Check sheet for the modelled part. Datum: model origin and axes. Units: mm. A direction names the side the tool comes from. Round coordinates to 2 decimals unless told otherwise and drop trailing zeros. Loops run counter-clockwise (first coordinate to the right, second up) from the corner with the lowest first, then second, coordinate; pieces in that order, holes last. Notation, with made-up numbers: (9.5, 20) -> (15.5, 20) arc R19 ccw to (15.5, 47) -> close; hole circle Ø7 at (87.25, -37). An arc over 180 degrees is marked (long way). One line per question, with ' | ' between items.
```python
from build123d import *

# Parameters (mm, degrees)
SKETCH1_W           = 29
SKETCH1_H           = 28
SKETCH1_W_2         = 25
SKETCH1_H_2         = 13
BOSS_EXTRUDE1_DEPTH = 2
SKETCH2_R           = 1.45
CUT_EXTRUDE1_DEPTH  = 3
BOSS_EXTRUDE2_DEPTH = 29
SKETCH5_W           = 29
SKETCH5_H           = 2
BOSS_EXTRUDE3_DEPTH = 1
SKETCH6_W           = 2
SKETCH6_H           = 33
SKETCH6_H_2         = 1.6
BOSS_EXTRUDE4_DEPTH = 3
SKETCH7_W           = 2
SKETCH7_H           = 33
SKETCH7_H_2         = 1.6
BOSS_EXTRUDE5_DEPTH = 3


with BuildPart() as part:
    # Sketch1 → Boss-Extrude1 (new body)
    with BuildSketch(Plane.XY):
        with Locations((0, -2)):
            Rectangle(SKETCH1_W, SKETCH1_H)
        Rectangle(SKETCH1_W_2, SKETCH1_H_2, mode=Mode.SUBTRACT)
    extrude(amount=BOSS_EXTRUDE1_DEPTH)

    # Sketch2 → Cut-Extrude1 (cut, through all)
    with BuildSketch(Plane.XY.offset(2)):
        with Locations((-12, 10.5)):
            Circle(SKETCH2_R)
        with Locations((-12, -13.5)):
            Circle(SKETCH2_R)
        with Locations((12, -13.5)):
            Circle(SKETCH2_R)
        with Locations((12, 10.5)):
            Circle(SKETCH2_R)
    extrude(amount=-CUT_EXTRUDE1_DEPTH, mode=Mode.SUBTRACT)

    # Sketch3 → Boss-Extrude2 (add, through all)
    with BuildSketch(Plane(origin=(14.5, 0, 0), x_dir=(0, 0, -1), z_dir=(1, 0, 0))):
        Polygon((-4, -20), (0, -20), (0, -18.4), (0, -16), (-2, -16), (-2, -18.4), (-4, -18.4), align=None)
    extrude(amount=-BOSS_EXTRUDE2_DEPTH)

    # Sketch5 → Boss-Extrude3 (add)
    with BuildSketch(Plane(origin=(0, 12, 0), x_dir=(1, 0, 0), z_dir=(0, 1, 0))):
        with Locations((0, -1)):
            Rectangle(SKETCH5_W, SKETCH5_H)
    extrude(amount=BOSS_EXTRUDE3_DEPTH)

    # Sketch6 → Boss-Extrude4 (add)
    with BuildSketch(Plane.ZY.offset(14.5)):
        with Locations((1, -3.5)):
            Rectangle(SKETCH6_W, SKETCH6_H)
        with Locations((3, -19.2)):
            Rectangle(SKETCH6_W, SKETCH6_H_2)
    extrude(amount=BOSS_EXTRUDE4_DEPTH)

    # Sketch7 → Boss-Extrude5 (add)
    with BuildSketch(Plane(origin=(14.5, 0, 0), x_dir=(0, 0, -1), z_dir=(1, 0, 0))):
        with Locations((-1, -3.5)):
            Rectangle(SKETCH7_W, SKETCH7_H)
        with Locations((-3, -19.2)):
            Rectangle(SKETCH7_W, SKETCH7_H_2)
    extrude(amount=BOSS_EXTRUDE5_DEPTH)


solid = part.part
```
(1) Go/stop test with flat-tipped pins: pin 1 (4.5 mm diameter, centred on x = 12, y = -13.5, fed in from -Z); pin 2 (2.5 mm diameter, centred on x = -12, y = -13.5, fed in from +Z). Record where each tip stops, or that it passes through.
Answer:
pin 1: stops at z = 0 | pin 2: passes through
(2) Sectioned sample at D-D, the plane x = -0.5. Record the cut outline in (y, z).
Answer:
outline: (-20, 0) -> (-6.5, 0) -> (-6.5, 2) -> (-18.4, 2) -> (-18.4, 4) -> (-20, 4) -> close; (6.5, 0) -> (13, 0) -> (13, 2) -> (6.5, 2) -> close
(3) Scan lines: probe 1 along Y at (x, z) = (-12, 0.65); probe 2 along Y at (x, z) = (3, 1); probe 3 along X at (y, z) = (6, 0.3). Record each from-to range of solid material in increasing order.
Answer:
probe 1: y = -20 to -14.95, -12.05 to -6.5, 6.5 to 9.05, 11.95 to 13 | probe 2: y = -20 to -6.5, 6.5 to 13 | probe 3: x = -17.5 to -12.5, 12.5 to 17.5
(4) Sectioned sample at A-A, the plane x = -11. Record the cut outline in (y, z), and give its area (3 significant figures).
Answer:
outline: (-20, 0) -> (-14.55, 0) -> (-14.55, 2) -> (-18.4, 2) -> (-18.4, 4) -> (-20, 4) -> close; (-12.45, 0) -> (-6.5, 0) -> (-6.5, 2) -> (-12.45, 2) -> close; (6.5, 0) -> (9.45, 0) -> (9.45, 2) -> (6.5, 2) -> close; (11.55, 0) -> (13, 0) -> (13, 2) -> (11.55, 2) -> close | area: 34.8 mm2
(5) Mould release check, pull along Y, two halves, no side actions. Record for faces 4 (the face through (0, -20, 2)), 5 (the face through (-12.5, 0, 1)), 6 (the face through (0, -7, 0)), 7 (the face through (0, -18.4, 3)): +Y half, -Y half, draft (parallel to the pull), parting line (faces both ways), or undercut.
Answer:
face 4: -Y half | face 5: undercut | face 6: draft | face 7: +Y half
(6) Sectioned sample at B-B, the plane y = 10.5. Record the cut outline in (x, z).
Answer:
outline: (-17.5, 0) -> (-13.45, 0) -> (-13.45, 2) -> (-17.5, 2) -> close; (-10.55, 0) -> (10.55, 0) -> (10.55, 2) -> (-10.55, 2) -> close; (13.45, 0) -> (17.5, 0) -> (17.5, 2) -> (13.45, 2) -> close
(7) Sectioned sample at C-C, the plane z = 1.45. Record the cut outline in (x, y), and give its area (3 significant figures).
Answer:
outline: (-17.5, -20) -> (17.5, -20) -> (17.5, 13) -> (-17.5, 13) -> close; hole circle Ø2.9 at (-12, -13.5); hole circle Ø2.9 at (-12, 10.5); hole (-12.5, -6.5) -> (12.5, -6.5) -> (12.5, 6.5) -> (-12.5, 6.5) -> close; hole circle Ø2.9 at (12, -13.5); hole circle Ø2.9 at (12, 10.5) | area: 804 mm2
(8) Set-up check for faces 1 (the face through (0, 6.5, 1)), 2 (the face through (0, -10, 2)), 3 (the face through (17.5, -3, 1)): record each of +Z, -Z, +X, -X, +Y, -Y from which the full face is reachable in a straight line by a thin tool's end or side.
Answer:
face 1: +Z, -Z | face 2: +Z, +X, -X, +Y | face 3: +Z, -Z, +X, +Y, -Y
